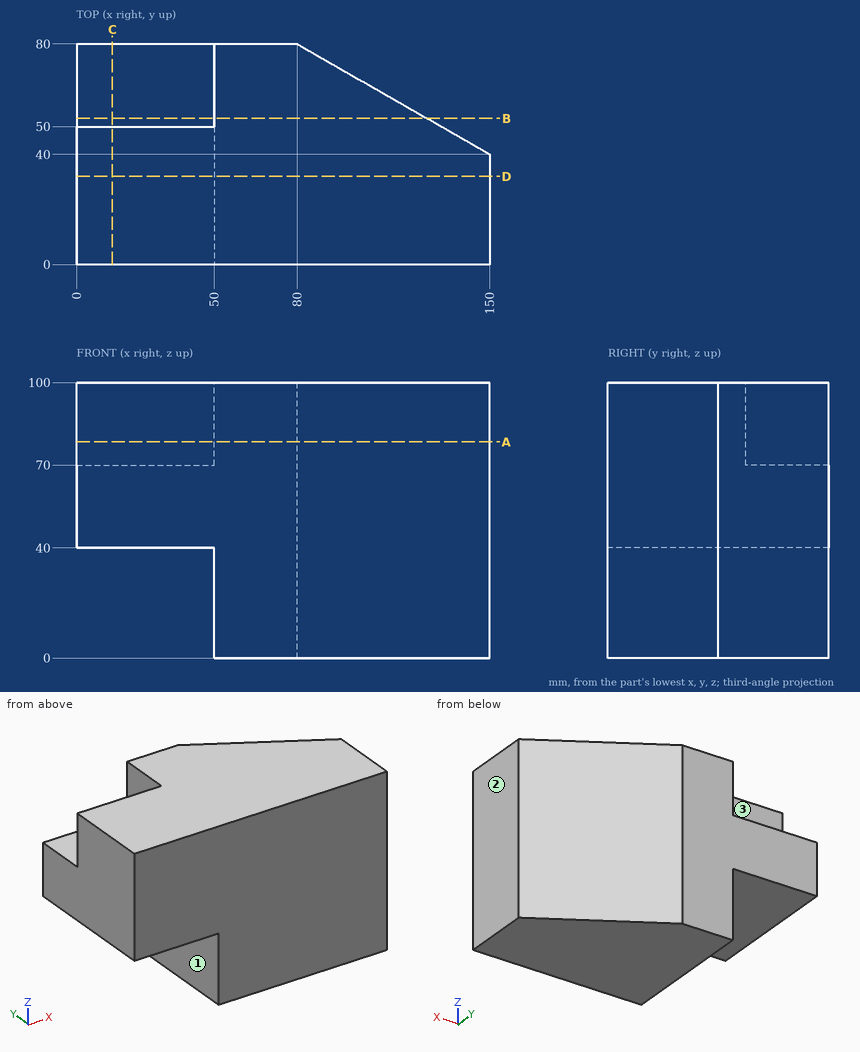
Print and shaded views of the part. All mm, measured from the part's lowest x, y and z. A direction names the side the tool comes from. Give positions to 0.01 mm unless a question says otherwise; leave off trailing zeros. Loops run counter-clockwise (first coordinate to the right, second up) from the corner with the lowest first, then second, coordinate; pieces in that order, holes last. Notation, with made-up numbers: (72.5, 73) -> (122.5, 73) arc R30 ccw to (122.5, 109) -> close; hole circle Ø7 at (-24, 68.5). An arc over 180 degrees is marked (long way). Use a Markdown table: item, result.
1. Slice it at C-C (x = 13). List the corners of the cut face in (y, z), plus the area to 3 significant figures.
Check result:
| item | result |
|---|---|
| outline | (0, 40) -> (80, 40) -> (80, 70) -> (50, 70) -> (50, 100) -> (0, 100) -> close |
| area | 3,900 mm^2 |
2. Wall check: L1, parallel to Z at x = 10, y = 47.5; L2, parallel to Z at x = 45, y = 74; L3, parallel to Y at x = 22, z = 89. Give the ranges that are in metal, low to high. Write a range as [from, to].
Check result:
| item | result |
|---|---|
| L1 | z = [40, 100] |
| L2 | z = [40, 70] |
| L3 | y = [0, 50] |
3. Slice it at A-A (z = 78.5). List the corners of the cut face in (x, y).
Check result:
| item | result |
|---|---|
| outline | (0, 0) -> (150, 0) -> (150, 40) -> (80, 80) -> (50, 80) -> (50, 50) -> (0, 50) -> close |
4. Slice it at D-D (y = 32). List the corners of the cut face in (x, z), plus the area to 3 significant figures.
Check result:
| item | result |
|---|---|
| outline | (0, 40) -> (50, 40) -> (50, 0) -> (150, 0) -> (150, 100) -> (0, 100) -> close |
| area | 13,000 mm^2 |
5. Slice it at B-B (y = 53). List the corners of the cut face in (x, z).
Check result:
| item | result |
|---|---|
| outline | (0, 40) -> (50, 40) -> (50, 0) -> (127.25, 0) -> (127.25, 100) -> (50, 100) -> (50, 70) -> (0, 70) -> close |
6. Flat gauge pins, fed straight in: pin 1 (10 mm diameter, centred on y = 67, z = 14, fed in from -X); pin 2 (6 mm diameter, centred on x = 124, z = 35.5, fed in from +Y); pin 3 (10 mm diameter, centred on y = 46.5, z = 39.5, fed in from +X) (3 decimals). Where does each tip first touch, or does it go through?
Check result:
| item | result |
|---|---|
| pin 1 | stops at x = 50 |
| pin 2 | stops at y = 56.57 |
| pin 3 | stops at x = 147.375 |
7. Which spindle directions (+Z, -Z, +X, -X, +Y, -Y) get a long thin tool onto all of the face, cutting with end or side? Do the marked faces 1, 2 and 3. Say none if no direction does.
Check result:
| item | result |
|---|---|
| face 1 | -Z, -X, +Y, -Y |
| face 2 | +Z, -Z, +X, +Y, -Y |
| face 3 | +Z, -X, +Y |
